```python
from build123d import *

# Parameters (mm, degrees)
SKETCH1_W           = 5.7
SKETCH1_H           = 4
SKETCH1_W_2         = 3.6
SKETCH1_H_2         = 2.4
BOSS_EXTRUDE1_DEPTH = 3.7
CHAMFER1_SIZE       = 0.4


with BuildPart() as part:
    # Sketch1 → Boss-Extrude1 (new body)
    with BuildSketch(Plane.XY):
        Rectangle(SKETCH1_W, SKETCH1_H)
        with Locations((0, 3.2)):
            Rectangle(SKETCH1_W_2, SKETCH1_H_2)
    extrude(amount=BOSS_EXTRUDE1_DEPTH)

    # Chamfer1
    chamfer1_edges = [part.edges().sort_by_distance(p)[0] for p in [
        (-1.8, 4.4, 1.85),
        (1.8, 4.4, 1.85),
    ]]
    chamfer(chamfer1_edges, length=CHAMFER1_SIZE)


solid = part.part
```
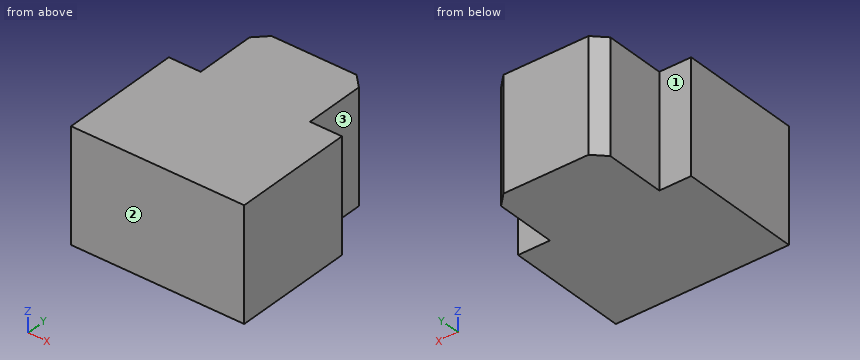
Could you check a few things on this model? Use its own coordinates, in mm. Face numbers are marked on the shaded views. A direction names the side the tool comes from. Round coordinates to 2 decimals unless told otherwise and drop trailing zeros. Loops run counter-clockwise (first coordinate to the right, second up) from the corner with the lowest first, then second, coordinate; pieces in that order, holes last. Notation, with made-up numbers: M -7.75,57 L 17.25,57 A17 ccw 17.25,72 Z; hole C 26,18 d4. An arc over 180 degrees is marked long. Write item = value, one per line.
1. I want a section at A-A, the plane z = 0.55. Write out the boundary of the cut face in (x, y).
Results below:
outline = M -2.85,-2 L 2.85,-2 L 2.85,2 L 1.8,2 L 1.8,4 L 1.4,4.4 L -1.4,4.4 L -1.8,4 L -1.8,2 L -2.85,2 Z
2. Will these pins go through, and if not, where does the flat tip stop? P1, Ø2, axis at y = 3.5, z = 2.5, coming from the +X side; P2, Ø0.5, axis at x = 2, z = 1, coming from the +Y side.
Results below:
P1 = 1.8
P2 = 4.05
3. Which directions (+Z, -Z, +X, -X, +Y, -Y) give clear straight access to the entire face, cutting with the end or side of a thin tool? Please do the marked faces 1, 2 and 3.
Results below:
face_1 = +Z, -Z, -X, +Y
face_2 = +Z, -Z, +X, -X, -Y
face_3 = +Z, -Z, +X, +Y
4. I want a section at C-C, the plane y = 2.75. Write out the boundary of the cut face in (x, z).
Results below:
outline = M -1.8,0 L 1.8,0 L 1.8,3.7 L -1.8,3.7 Z
5. I need wall thicknesses on probe 1 along Y at (x, z) = (2.5, 2.55); probe 2 along X at (y, z) = (3.75, 2); probe 3 along Y at (x, z) = (-1.7, 2.45). Which ranges of each line are inside material? Lowest first, please.
Results below:
probe_1 = -2 to 2
probe_2 = -1.8 to 1.8
probe_3 = -2 to 4.1
6. I want a section at B-B, the plane x = -1.6. Write out the boundary of the cut face in (y, z), and give its area (3 significant figures).
Results below:
outline = M -2,0 L 4.2,0 L 4.2,3.7 L -2,3.7 Z
area = 22.9 mm²
